from build123d import *

# Parameters (mm, degrees)
SKETCH1_W           = 27.5
SKETCH1_H           = 23
BOSS_EXTRUDE1_DEPTH = 2.7
SKETCH2_W           = 12
SKETCH2_H           = 8
CUT_EXTRUDE1_DEPTH  = 3.7
SKETCH4_W           = 24
SKETCH4_H           = 10.05
BOSS_EXTRUDE4_DEPTH = 5
BOSS_EXTRUDE4_TAPER = 20
SKETCH3_W           = 13
SKETCH3_H           = 7.5
CUT_EXTRUDE3_DEPTH  = 7.7


with BuildPart() as part:
    # Sketch1 → Boss-Extrude1 (new body)
    with BuildSketch(Plane(origin=(0, 0, 0), x_dir=(0, 0, -1), z_dir=(1, 0, 0))):
        Rectangle(SKETCH1_W, SKETCH1_H)
    extrude(amount=-BOSS_EXTRUDE1_DEPTH)

    # Sketch2 → Cut-Extrude1 (cut, through all)
    with BuildSketch(Plane(origin=(0, 0, 0), x_dir=(0, 0, -1), z_dir=(1, 0, 0))):
        with Locations((0, 7.5)):
            Rectangle(SKETCH2_W, SKETCH2_H)
    extrude(amount=-CUT_EXTRUDE1_DEPTH, mode=Mode.SUBTRACT)

    # Sketch4 → Boss-Extrude4 (add)
    with BuildSketch(Plane.ZY.offset(2.7)):
        with Locations((0, -5.025)):
            Rectangle(SKETCH4_W, SKETCH4_H)
    extrude(amount=BOSS_EXTRUDE4_DEPTH, taper=BOSS_EXTRUDE4_TAPER)

    # Sketch3 → Cut-Extrude3 (cut)
    with BuildSketch(Plane(origin=(0, 0, 0), x_dir=(0, 0, -1), z_dir=(1, 0, 0))):
        with Locations((0, -5.75)):
            Rectangle(SKETCH3_W, SKETCH3_H)
    extrude(amount=-CUT_EXTRUDE3_DEPTH, mode=Mode.SUBTRACT)


solid = part.part
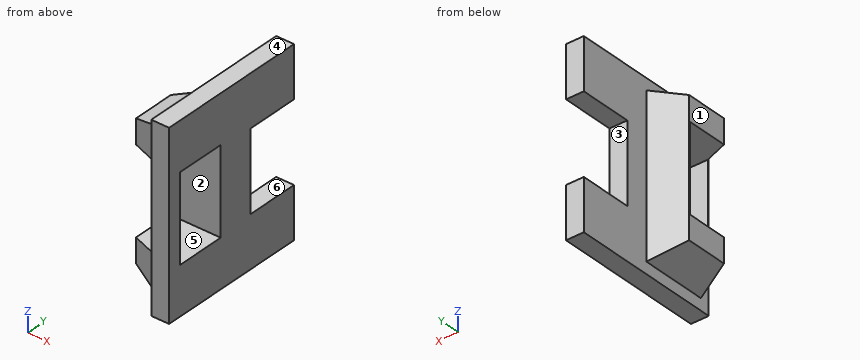
CAD build for the part. Positions are in the model's coordinates, mm. Face numbers are marked on the shaded views. A direction names the side the tool comes from. Give positions to 0.01 mm unless a question says otherwise; leave off trailing zeros. Loops run counter-clockwise (first coordinate to the right, second up) from the corner with the lowest first, then second, coordinate; pieces in that order, holes last. Notation, with made-up numbers: M -33.5,16.5 L -15.5,16.5 A27 ccw -15.5,53.5 Z; hole C 69,12.25 d3. An arc over 180 degrees is marked long. Answer in a Markdown table with one row per item. Add a question column.
Item 1: Drop flat-ended pins along their axis: P1, Ø1, axis at x = -5, z = -8.5, coming from the -Y side; P2, Ø1.3, axis at x = -1.5, z = 3, coming from the +Y side; P3, Ø3, axis at x = -6.5, y = -5.5, coming from the +Z side. Give the stop position or say it passes through.
Item 2: Tool access for the marked faces 4, 5 and 6: list every direction of +Z, -Z, +X, -X, +Y, -Y with a clear straight run to the whole face (end or side of a thin tool).
Item 3: Band-saw the part on A-A on x = -1.5. Give the cut face in (y, z).
Item 4: Probe probe 1 along Y at (x, z) = (-2.25, 1.75); probe 2 along Z at (x, y) = (-2.25, -3.25); probe 3 along X at (y, z) = (5.75, 7.75). List the from-to ranges inside material, lowest first.
Item 5: Mould opens along Y. For the marked faces 1, 2 and 3 say: +Y half, -Y half, draft (parallel to the pull), parting line (faces both ways), or undercut.
Item 6: Band-saw the part on B-B on y = 4. Give the cut face in (x, z).
Reply:
| question | item | result |
|---|---|---|
| 1 | P1 | stops at y = -9.39 |
| 1 | P2 | stops at y = 3.5 |
| 1 | P3 | stops at z = 11.16 |
| 2 | face 4 | +Z, +X, -X, +Y, -Y |
| 2 | face 5 | +X, -X |
| 2 | face 6 | +X, -X, +Y |
| 3 | outline | M -11.5,-13.75 L 11.5,-13.75 L 11.5,-6 L 3.5,-6 L 3.5,6 L 11.5,6 L 11.5,13.75 L -11.5,13.75 Z; hole M -9.5,-6.5 L -2,-6.5 L -2,6.5 L -9.5,6.5 Z |
| 4 | probe 1 | y = -11.5 to -9.5, -2 to 3.5 |
| 4 | probe 2 | z = -13.75 to -6.5, 6.5 to 13.75 |
| 4 | probe 3 | x = -2.7 to 0 |
| 5 | face 1 | draft |
| 5 | face 2 | undercut |
| 5 | face 3 | +Y half |
| 6 | outline | M -2.7,-13.75 L 0,-13.75 L 0,-6 L -2.7,-6 Z; M -2.7,6 L 0,6 L 0,13.75 L -2.7,13.75 Z |
